Study the drawing (mm; zero at the part's minimum x, y, z) and answer. A direction names the side the tool comes from. Coordinates: 2 decimals unless noted, no trailing zeros. Loops run counter-clockwise (first coordinate to the right, second up) from the corner with the lowest first, then second, coordinate; pieces in that order, holes last. Notation, with made-up numbers: M -6,31 L 30,31 A17 ccw 30,41 Z; hole C -30.75,26.5 d9. An arc over 180 degrees is marked long. Use one line per item in the form item = value. Start each with the question number.
1. The part is cut by section C-C (z = 22.25). Give the vertices of the cut face in (x, y) (3 decimals).
2. A tool of negligible diameter and unlimited length cuts with its end or side. For the marked faces 1 and 2, from which of +Z, -Z, +X, -X, +Y, -Y can it reach the whole face along a straight path? Write none if from no direction.
3. The part is cut by section B-B (z = 4). Give the vertices of the cut face in (x, y).
4. The part is cut by section A-A (x = 4). Give the vertices of the cut face in (y, z).
5. Flat-ended cylindrical pins translate along their axes: pin 1 (4 mm diameter, centred on x = 1.5, z = 14, fed in from -Y); pin 2 (1.5 mm diameter, centred on y = 5.5, z = 11, fed in from +X); pin 3 (2 mm diameter, centred on y = 5.5, z = 3.5, fed in from -X). Find the tip coordinate at first contact, or state that the pin passes through.
6. Find the intervals of material crossed by probe 1 along X at (y, z) = (2, 9.5); probe 2 along X at (y, z) = (5, 17); probe 3 along Y at (x, z) = (1.5, 22.75), in increasing order. Write a range as [from, to].
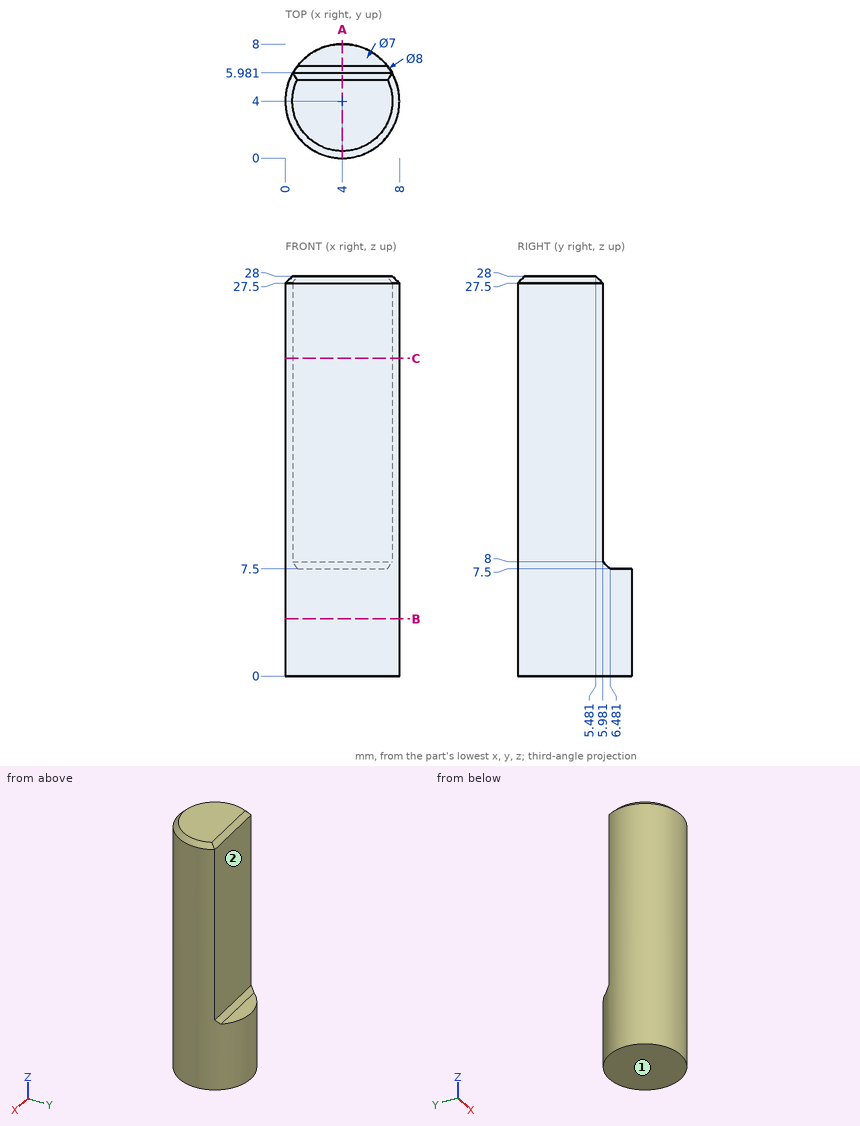
Computed values:
q1.outline = M 0.525,5.981 A4 ccw long 7.475,5.981 Z
q2.face_1 = -Z, +X, -X, +Y, -Y
q2.face_2 = +Z, +X, -X, +Y
q3.outline = C 4,4 d8
q4.outline = M 0,0 L 8,0 L 8,7.5 L 6.48,7.5 L 5.98,8 L 5.98,27.5 L 5.48,28 L 0.5,28 L 0,27.5 Z
q5.pin_1 = 0.03
q5.pin_2 = 7.93
q5.pin_3 = 0.03
q6.probe_1 = [0.54, 7.46]
q6.probe_2 = [0.13, 7.87]
q6.probe_3 = [0.88, 5.98]
